Could you check a few things on this model? Use its own coordinates, in mm. Face numbers are marked on the shaded views. A direction names the side the tool comes from. Give positions to 0.01 mm unless a question says otherwise; leave off trailing zeros. Order: outer loops, then holes, each group sorted by start corner. A loop starts at its lowest first (then second) coordinate and runs counter-clockwise, first axis right, second up. Notation, with made-up numbers: (17.25, 13) - (37.25, 13) arc R24 cw to (37.25, 46) - close; hole circle Ø6 at (-30.75, 10.25). An arc over 180 degrees is marked (long way). Put each result on its own line as item: value.
Autodesk Inventor part; units mm, degrees
ref_plane "YZ Plane" through (0, 0, 0) normal (1, 0, 0) x (0, 1, 0)
ref_plane "XZ Plane" through (0, 0, 0) normal (0, 1, 0) x (-1, 0, 0)
ref_plane "XY Plane" through (0, 0, 0) normal (0, 0, 1) x (1, 0, 0)
sketch "Эскиз1" plane through (0, 0, 0) normal (0, 0, 1) x (1, 0, 0)
  line L0 (0, 0) -> (0, 35)
  line L1 (0, 35) -> (39, 35)
  line L2 (39, 35) -> (39, 27)
  line L3 (39, 27) -> (20, 27)
  line L4 (20, 27) -> (20, 0)
  line L5 (20, 0) -> (0, 0)
  dimension "d0" = 78
  dimension "d1" = 40
  dimension "d2" = 8
  dimension "d3" = 35
revolve "Вращение1" add sketch "Эскиз1" angle 360 about axis through (0, 0, 0) along (0, 1, 0)
sketch "Эскиз2" plane through (0, 35, 0) normal (0, 1, 0) x (1, 0, 0)
  circle A0 centre (0, 0) radius 39
  line L0 (-39, 0) -> (39, 0) construction
  line L1 (-27.6541, 27.5) -> (27.6541, 27.5)
  line L2 (-27.6541, -27.5) -> (27.6541, -27.5)
  line L3 (-25, -16) -> (25, -16) construction
  line L4 (25, -16) -> (25, 16) construction
  line L5 (25, 16) -> (-25, 16) construction
  line L6 (-25, 16) -> (-25, -16) construction
  line L7 (-25, -16) -> (25, 16) construction
  line L8 (25, -16) -> (-25, 16) construction
  circle A1 centre (-25, 16) radius 4.5
  circle A2 centre (-25, -16) radius 4.5
  circle A3 centre (25, -16) radius 4.5
  circle A4 centre (25, 16) radius 4.5
  dimension "d5" = 55
  dimension "d6" = 50
  dimension "d7" = 32
  dimension "d10" = 9
extrude "Выдавливание1" cut sketch "Эскиз2" against normal through all contours L1 A0 | A0 L2 | A1 | A2 | A3 | A4
hole "Отверстие1" at (0, 35, 0) direction (0, -1, 0) diameter 16 end through all
chamfer "Фаска1" distance 3 angle 45 1 edges at (0, 0, -8)
chamfer "Фаска2" distance 2 angle 45 1 edges at (-20, 0, 0)
properties part number "Втулка 4"
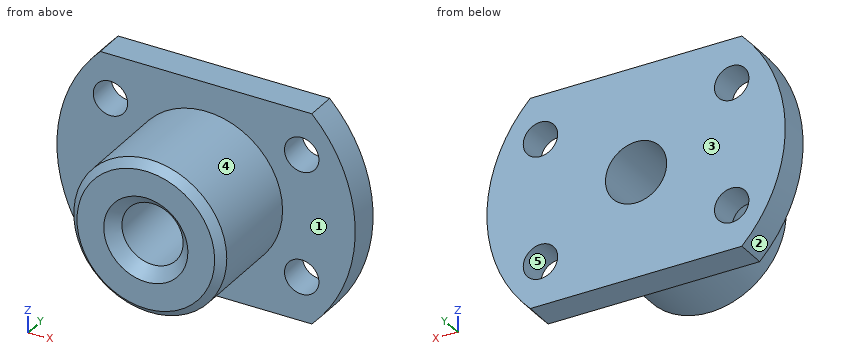
1) If I drill on line 1 (Z direction, x = 25, y = 29.75); line 2 (X direction, y = 30.5, z = 16); line 3 (Y direction, x = 2, z = 25), over which ranges is the centre line in solid material (lowest first)? Write a range as [from, to].
Filled in:
line 1: z = [-27.5, -20.5], [-11.5, 11.5], [20.5, 27.5]
line 2: x = [-35.57, -29.5], [-20.5, 20.5], [29.5, 35.57]
line 3: y = [27, 35]
2) Suppose I cut it at D-D, the plane x = 0. List the corners of the cut face in (y, z) for me, and give its area (3 significant figures).
Filled in:
outline: (0, -18) - (2, -20) - (27, -20) - (27, -27.5) - (35, -27.5) - (35, -8) - (3, -8) - (0, -11) - close; (0, 11) - (3, 8) - (35, 8) - (35, 27.5) - (27, 27.5) - (27, 20) - (2, 20) - (0, 18) - close
area: 947 mm^2
3) Which directions (+Z, -Z, +X, -X, +Y, -Y) give clear straight access to the entire face, cutting with the end or side of a thin tool? Please do the marked faces 1 and 2.
Filled in:
face 1: -Y
face 2: -X, +Y, -Y
4) Suppose I cut it at C-C, the plane y = 29. List the corners of the cut face in (x, z) for me.
Filled in:
outline: (-27.65, -27.5) - (27.65, -27.5) arc R39 ccw to (27.65, 27.5) - (-27.65, 27.5) arc R39 ccw to start; hole circle Ø9 at (-25, -16); hole circle Ø9 at (-25, 16); hole circle Ø16 at (0, 0); hole circle Ø9 at (25, -16); hole circle Ø9 at (25, 16)
5) Suppose I cut it at A-A, the plane x = -25. List the corners of the cut face in (y, z) for me, and give its area (3 significant figures).
Filled in:
outline: (27, -27.5) - (35, -27.5) - (35, -20.5) - (27, -20.5) - close; (27, -11.5) - (35, -11.5) - (35, 11.5) - (27, 11.5) - close; (27, 20.5) - (35, 20.5) - (35, 27.5) - (27, 27.5) - close
area: 296 mm^2
6) Suppose I cut it at B-B, the plane z = 0. List the corners of the cut face in (x, y) for me.
Filled in:
outline: (-39, 27) - (-20, 27) - (-20, 2) - (-18, 0) - (-11, 0) - (-8, 3) - (-8, 35) - (-39, 35) - close; (8, 3) - (11, 0) - (18, 0) - (20, 2) - (20, 27) - (39, 27) - (39, 35) - (8, 35) - close
7) We'd pull the mould along Z, two halves only. Please class the marked faces 3, 4 and 5: pulls with the +Z half, pulls with the -Z half, needs draft (parallel to the pull), parting line crosses it, or undercut.
Filled in:
face 3: needs draft
face 4: parting line crosses it
face 5: undercut
8) I'm going to push flat-ended pins straight in: pin 1 (3 mm diameter, centred on x = -8, y = 18, fed in from +Z); pin 2 (5 mm diameter, centred on y = 21, z = 1.5, fed in from -X); pin 3 (4 mm diameter, centred on x = -13, y = 21, fed in from +Z). Where does each tip first touch, or does it pass through?
Filled in:
pin 1: stops at z = 18.91
pin 2: stops at x = -20
pin 3: stops at z = 16.7
